Autodesk Inventor part; units mm, degrees
ref_plane "YZ Plane" through (0, 0, 0) normal (1, 0, 0) x (0, 1, 0)
ref_plane "XZ Plane" through (0, 0, 0) normal (0, 1, 0) x (-1, 0, 0)
ref_plane "XY Plane" through (0, 0, 0) normal (0, 0, 1) x (1, 0, 0)
sketch "Эскиз1" plane through (0, 0, 0) normal (0, 1, 0) x (-1, 0, 0)
  circle A0 centre (0, 0) radius 4.45
  circle A1 centre (0, 0) radius 5.45
  line L0 (0, 0) -> (4.349, 3.2846)
  line L1 (0, 0) -> (4.349, -3.2846)
  point P0 (3.551, -2.6819)
  point P1 (3.551, 2.6819)
  dimension "d0" = 8.9
  dimension "d1" = 10.9
extrude "Выдавливание1" add sketch "Эскиз1" along normal blind 30 contours A0 L1 A1 L0 picked at (-3.4029, -3.7722)
sketch "Эскиз2" plane through (0, 30, 0) normal (0, 1, 0) x (1, 0, 0)
  arc A0 (-3.551, -2.6819) -> (-4.4437, -2.1521) centre (-6.2523, -6.2159) ccw
  arc A1 (-4.4437, -2.1521) -> (-5.6006, -3.9578) centre (-4.878, -3.1473) ccw
  line L0 (-5.6006, -3.9578) -> (-4.9293, -3.1033)
  arc A2 (-4.3504, -3.2701) -> (-4.9293, -3.1033) centre (-4.7187, -3.4605) ccw
  line L1 (-3.551, -2.6819) -> (-4.349, -3.2846)
  line L2 (-4.349, -3.2846) -> (-3.551, -2.6819)
  line L3 (-4.349, -3.2846) -> (-4.3504, -3.2701)
  line L4 (-0.0151, 0) -> (-3.489, 0)
  arc A3 (-4.4437, 2.1521) -> (-3.551, 2.6819) centre (-6.2523, 6.2159) ccw
  arc A4 (-4.9293, 3.1033) -> (-4.3504, 3.2701) centre (-4.7187, 3.4605) ccw
  line L5 (-3.551, 2.6819) -> (-4.349, 3.2846)
  line L6 (-4.349, 3.2846) -> (-3.551, 2.6819)
  line L7 (-4.349, 3.2846) -> (-4.3504, 3.2701)
  arc A5 (-5.6006, 3.9578) -> (-4.4437, 2.1521) centre (-4.878, 3.1473) ccw
  line L8 (-5.6006, 3.9578) -> (-4.9293, 3.1033)
  point P0 (-3.551, 2.6819)
  point P1 (-4.349, -3.2846)
  point P2 (-5.3694, -4.0591)
  point P3 (-4.349, 3.2846)
  point P4 (-5.3694, 4.0591)
  point P5 (-4.349, 3.2846)
  dimension "d25" = 1.0859
sketch "Эскиз3" plane through (0, 30, 0) normal (0, 1, 0) x (1, 0, 0)
  arc A0 (-4.349, -3.2846) -> (-4.349, 3.2846) centre (0, 0) ccw
  line L0 (11.5, -6.95) -> (11.5, 6.95)
  arc A1 (-3.551, -2.6819) -> (-3.551, 2.6819) centre (0, 0) ccw
  line L1 (0, -5.45) -> (0, -4.45)
  line L2 (0, 4.45) -> (0, 5.45)
  line L3 (11.5, 6.95) -> (11.5, 10.95)
  line L4 (11.5, -6.95) -> (11.5, -10.95)
  line L5 (0, 0.95) -> (0, 5.45)
  line L6 (11.5, -10.95) -> (0, -10.95)
  line L7 (0, -10.95) -> (0, -5.45)
  line L8 (11.5, 10.95) -> (0, 10.95)
  line L9 (0, 10.95) -> (0, 5.45)
  arc A2 (0, -4.45) -> (0, 4.45) centre (0, 0) ccw
  dimension "d13" = 4
  dimension "d14" = 4
  dimension "d22" = 21.9
  dimension "d23" = 6.5
extrude "Выдавливание3" add sketch "Эскиз3" against normal blind 30
ref_plane "РабПлоскость1" through (11.5, 20, 4.95) normal (1, 0, 0) x (0, 0, -1)
sketch "Эскиз4" plane through (11.5, 20, 4.95) normal (1, 0, 0) x (0, 0, -1)
  line L0 (4.95, -20) -> (4.95, 10)
  line L1 (1, 10) -> (8.9, 10)
  circle A0 centre (4.95, -12) radius 5
  line L2 (14.4, -20) -> (-4.5, -20)
  circle A1 centre (4.95, 2) radius 5
  line L3 (-4.5, 10) -> (14.4, 10)
  point P0 (7.3306, 10)
  point P1 (2.5694, 10)
  point P2 (4.95, 10)
  dimension "d15" = 10
  dimension "d16" = 8
  dimension "d17" = 10
  dimension "d18" = 8
extrude "Выдавливание4" cut sketch "Эскиз4" against normal blind 2
extrude "Выдавливание5" add sketch "Эскиз2" against normal blind 30
sketch "Эскиз5" plane through (0, 30, 0) normal (0, 1, 0) x (1, 0, 0)
  arc A0 (0, 5.45) -> (-4.349, 3.2846) centre (0, 0) ccw
  line L0 (-4.349, 3.2846) -> (-4.3504, 3.2701)
  arc A1 (-4.9293, 3.1033) -> (-4.3504, 3.2701) centre (-4.7187, 3.4605) ccw
  line L1 (-4.9293, 3.1033) -> (-5.6006, 3.9578)
  arc A2 (-5.6006, 3.9578) -> (-4.4437, 2.1521) centre (-4.878, 3.1473) ccw
  arc A3 (-4.4437, 2.1521) -> (-3.551, 2.6819) centre (-6.2523, 6.2159) ccw
  arc A4 (-3.551, -2.6819) -> (-3.551, 2.6819) centre (0, 0) ccw
  arc A5 (-3.551, -2.6819) -> (-4.4437, -2.1521) centre (-6.2523, -6.2159) ccw
  arc A6 (-4.4437, -2.1521) -> (-5.6006, -3.9578) centre (-4.878, -3.1473) ccw
  line L2 (-5.6006, -3.9578) -> (-4.9293, -3.1033)
  arc A7 (-4.3504, -3.2701) -> (-4.9293, -3.1033) centre (-4.7187, -3.4605) ccw
  line L3 (-4.3504, -3.2701) -> (-4.349, -3.2846)
  arc A8 (-4.349, -3.2846) -> (0, -5.45) centre (0, 0) ccw
  line L4 (0, -5.45) -> (0, -10.95)
  line L5 (0, -10.95) -> (11.5, -10.95)
  line L6 (11.5, -10.95) -> (11.5, 10.95)
  line L7 (11.5, 10.95) -> (0, 10.95)
  line L8 (0, 10.95) -> (0, 5.45)
  line L9 (0, 4.45) -> (0, 5.45)
  line L10 (0, -4.45) -> (0, -5.45)
extrude "Выдавливание6" [suppressed]
sketch "Эскиз6" plane through (11.5, 30, 10.95) normal (1, 0, 0) x (0, 0, -1)
  arc A0 (15.95, -22) -> (15.95, -22) centre (10.95, -22) ccw
  arc A1 (15.95, -8) -> (15.95, -8) centre (10.95, -8) ccw
  point P0 (10.95, -30)
extrude "Выдавливание7" [suppressed]
properties part number "крепление маркера 9мм"
Could you check a few things on this model? Use its own coordinates, in mm. A direction names the side the tool comes from. Coordinates: 2 decimals unless noted, no trailing zeros. Write each loop counter-clockwise with the first axis right and the second up, starting at its lowest first coordinate (ties: lowest second). Pieces come first, ordered by that corner, then holes. Notation, with made-up numbers: (-28.75, 71.25) - (-0.75, 71.25) arc R31 ccw to (-0.75, 103.25) - close; hole circle Ø3 at (22.25, -32). An arc over 180 degrees is marked (long way). Write item = value, one per line.
1) Suppose I cut it at D-D on x = -4. Please give me the cut outline in (y, z), plus the area to 3 significant figures.
Result set:
outline = (0, -3.7) - (30, -3.7) - (30, -2.38) - (0, -2.38) - close; (0, 2.38) - (30, 2.38) - (30, 3.7) - (0, 3.7) - close
area = 79.3 mm2
2) Suppose I cut it at C-C on z = 0. Please give me the cut outline in (x, y), plus the area to 3 significant figures.
Result set:
outline = (4.45, 0) - (11.5, 0) - (11.5, 3) - (9.5, 3) - (9.5, 13) - (11.5, 13) - (11.5, 17) - (9.5, 17) - (9.5, 27) - (11.5, 27) - (11.5, 30) - (4.45, 30) - close
area = 172 mm2
3) We'd pull the mould along Z, two halves only. Please class faces 1 (the cylindrical face through (-2.461, 14.79, -4.863)), 2 (the cylindrical face through (10.51, 17.12, 1.08)), 3 (the flat face through (0, 15, 8)): +Z half, -Z half, draft (parallel to the pull), parting line (faces both ways), or undercut.
Result set:
face_1 = -Z half
face_2 = undercut
face_3 = draft
4) Will these pins go through, and if not, where does the flat tip stop? pin 1 Ø5 at (y, z) = (10, 1) entering from +X; pin 2 Ø6 at (y, z) = (15, 8.5) entering from -X; pin 3 Ø6 at (y, z) = (22, 0) entering from -X.
Result set:
pin_1 = 9.5
pin_2 = 0
pin_3 = -5.95
5) Suppose I cut it at B-B on x = 0.75. Please give me the cut outline in (y, z), plus the area to 3 significant figures.
Result set:
outline = (0, -10.95) - (30, -10.95) - (30, -4.39) - (0, -4.39) - close; (0, 4.39) - (30, 4.39) - (30, 10.95) - (0, 10.95) - close
area = 394 mm2
6) For faces 4 (the flat face through (-5.27, 15.21, -3.54)), 5 (the flat face through (9.5, 22, 0)), 6 (the flat face through (6, 15, -10.95)), 7 (the flat face through (-5.27, 15.21, 3.54)), 8 (the cylindrical face through (-3.98, 15.21, 2.39)), which set-ups out of +Z, -Z, +X, -X, +Y, -Y let a thin tool reach every point of the face, with its end or its side?
Result set:
face_4 = -Z, +Y, -Y
face_5 = +X
face_6 = -Z, +X, -X, +Y, -Y
face_7 = +Z, +Y, -Y
face_8 = +Y, -Y
7) Please list where these lines run through material, in increasing order: line 1 (Y direction, x = 10.55, z = 0); line 2 (Z direction, x = 10, y = 22); line 3 (Z direction, x = -0.25, y = 15.75). Write a range as [from, to].
Result set:
line_1 = [0, 3], [13, 17], [27, 30]
line_2 = [-10.95, -5], [5, 10.95]
line_3 = [-5.44, -4.44], [4.44, 5.44]
